Build history of the part. All positions in model axes, mm. A direction names the side the tool comes from. Round coordinates to 2 decimals unless told otherwise and drop trailing zeros. Write each loop counter-clockwise with the first axis right and the second up, starting at its lowest first coordinate (ties: lowest second). Pieces come first, ordered by that corner, then holes. Notation, with made-up numbers: (81.25, -8) -> (115.25, -8) arc R17 ccw to (115.25, -4) -> close; hole circle Ø4 at (-34.75, 88.25). An arc over 180 degrees is marked (long way). One line per question, with ' | ' between items.
from build123d import *

# Parameters (mm, degrees)
SKETCH1_W           = 75
SKETCH1_H           = 41
BOSS_EXTRUDE1_DEPTH = 4
SKETCH2_W           = 75
SKETCH2_H           = 2
BOSS_EXTRUDE2_DEPTH = 10
SKETCH3_W           = 75
SKETCH3_H           = 2
BOSS_EXTRUDE3_DEPTH = 10
SKETCH6_W           = 14.75
SKETCH6_H           = 20
CUT_EXTRUDE3_DEPTH  = 44.891912695
SKETCH7_W           = 75
SKETCH7_H           = 20
CUT_EXTRUDE4_DEPTH  = 1
SKETCH10_R          = 1.625
CUT_EXTRUDE5_DEPTH  = 2
SKETCH11_W          = 10.5
SKETCH11_H          = 5
CUT_EXTRUDE6_DEPTH  = 2.5


with BuildPart() as part:
    # Sketch1 → Boss-Extrude1 (new body)
    with BuildSketch(Plane(origin=(0, 0, 0), x_dir=(1, 0, 0), z_dir=(0, 1, 0))):
        Rectangle(SKETCH1_W, SKETCH1_H)
    extrude(amount=BOSS_EXTRUDE1_DEPTH)

    # Sketch2 → Boss-Extrude2 (add)
    with BuildSketch(Plane(origin=(0, 4, 0), x_dir=(1, 0, 0), z_dir=(0, 1, 0))):
        with Locations((0, 19.5)):
            Rectangle(SKETCH2_W, SKETCH2_H)
    extrude(amount=BOSS_EXTRUDE2_DEPTH)

    # Sketch3 → Boss-Extrude3 (add)
    with BuildSketch(Plane(origin=(0, 4, 0), x_dir=(1, 0, 0), z_dir=(0, 1, 0))):
        with Locations((0, -19.5)):
            Rectangle(SKETCH3_W, SKETCH3_H)
    extrude(amount=BOSS_EXTRUDE3_DEPTH)

    # Sketch6 → Cut-Extrude3 (cut, through all)
    with BuildSketch(Plane(origin=(0, 4, 0), x_dir=(1, 0, 0), z_dir=(0, 1, 0))):
        with Locations((0, 5)):
            Rectangle(SKETCH6_W, SKETCH6_H)
    extrude(amount=-CUT_EXTRUDE3_DEPTH, mode=Mode.SUBTRACT)

    # Sketch7 → Cut-Extrude4 (cut)
    with BuildSketch(Plane(origin=(0, 4, 0), x_dir=(1, 0, 0), z_dir=(0, 1, 0))):
        with Locations((0, 5)):
            Rectangle(SKETCH7_W, SKETCH7_H)
    extrude(amount=-CUT_EXTRUDE4_DEPTH, mode=Mode.SUBTRACT)

    # Sketch10 → Cut-Extrude5 (cut)
    with BuildSketch(Plane.XY.offset(20.5)):
        with Locations((-32.5, 9)):
            Circle(SKETCH10_R)
        with Locations((32.5, 9)):
            Circle(SKETCH10_R)
    extrude(amount=-CUT_EXTRUDE5_DEPTH, mode=Mode.SUBTRACT)

    # Sketch11 → Cut-Extrude6 (cut)
    with BuildSketch(Plane(origin=(0, 4, 0), x_dir=(1, 0, 0), z_dir=(0, 1, 0))):
        with Locations((-32.25, -11)):
            Rectangle(SKETCH11_W, SKETCH11_H)
        with Locations((32.25, -11)):
            Rectangle(SKETCH11_W, SKETCH11_H)
    extrude(amount=-CUT_EXTRUDE6_DEPTH, mode=Mode.SUBTRACT)


solid = part.part
(1) Wall check: line 1 (Z direction, x = -28, y = 13); line 2 (Y direction, x = -32.5, z = 19.7) (3 decimals); line 3 (Z direction, x = 0.5, y = 2.5). Give the ranges that are in metal, low to high. Write a range as from..to.
Calculated:
line 1: -20.5..-18.5, 18.5..20.5 | line 2: 0..7.375, 10.625..14 | line 3: -20.5..-15, 5..20.5
(2) Slice it at C-C (z = -4.5). Write the cut outline in (x, y) (3 decimals), then the cut area to 3 significant figures.
Calculated:
outline: (-37.5, 0) -> (-7.375, 0) -> (-7.375, 3) -> (-37.5, 3) -> close; (7.375, 0) -> (37.5, 0) -> (37.5, 3) -> (7.375, 3) -> close | area: 181 mm2
(3) 3-axis set-ups, long thin cutter, end or side, ignore diameter. For faces 4 (the flat face through (7.375, 2, -5)), 5 (the cylindrical face through (30.877, 9.071, 19.514)), 6 (the flat face through (32, 3, 8.5)): which of +Z, -Z, +X, -X, +Y, -Y reach the whole face in a straight line?
Calculated:
face 4: +Y, -Y | face 5: +Z | face 6: +X, +Y
(4) Mould opens along X. For faces 1 (the flat face through (27, 3, 11)), 2 (the flat face through (0, 3, 5)), 3 (the flat face through (-32, 3, 13.5)) say: pulls with the +X half, pulls with the -X half, needs draft (parallel to the pull), parting line crosses it, or undercut.
Calculated:
face 1: pulls with the +X half | face 2: undercut | face 3: needs draft
(5) Slice it at A-A (x = -32.5). Write the cut outline in (y, z) (3 decimals), then the cut area to 3 significant figures.
Calculated:
outline: (0, -20.5) -> (14, -20.5) -> (14, -18.5) -> (4, -18.5) -> (4, -15) -> (3, -15) -> (3, 5) -> (4, 5) -> (4, 8.5) -> (1.5, 8.5) -> (1.5, 13.5) -> (4, 13.5) -> (4, 18.5) -> (7.375, 18.5) -> (7.375, 20.5) -> (0, 20.5) -> close; (10.625, 18.5) -> (14, 18.5) -> (14, 20.5) -> (10.625, 20.5) -> close | area: 165 mm2
(6) Slice it at B-B (y = 11.75). Write the cut outline in (x, z), then the cut area to 3 significant figures.
Calculated:
outline: (-37.5, -20.5) -> (37.5, -20.5) -> (37.5, -18.5) -> (-37.5, -18.5) -> close; (-37.5, 18.5) -> (37.5, 18.5) -> (37.5, 20.5) -> (-37.5, 20.5) -> close | area: 300 mm2
(7) Drop flat-ended pins along their axis: pin 1 (5.5 mm diameter, centred on x = 32.5, z = 10.5, fed in from +Y); pin 2 (1.5 mm diameter, centred on x = -34.5, z = 11, fed in from +Y); pin 3 (1.2 mm diameter, centred on y = 3, z = 12, fed in from +X). Give the stop position or say it passes through.
Calculated:
pin 1: y = 4 | pin 2: y = 1.5 | pin 3: x = 27
(8) Slice it at D-D (x = -5). Write the cut outline in (y, z), then the cut area to 3 significant figures.
Calculated:
outline: (0, -20.5) -> (14, -20.5) -> (14, -18.5) -> (4, -18.5) -> (4, -15) -> (0, -15) -> close; (0, 5) -> (4, 5) -> (4, 18.5) -> (14, 18.5) -> (14, 20.5) -> (0, 20.5) -> close | area: 124 mm2
